Could you check a few things on this model? Use its own coordinates, in mm. Face numbers are marked on the shaded views. Round coordinates to 2 decimals unless told otherwise and drop trailing zeros. Answer in a Markdown table with one row per item.
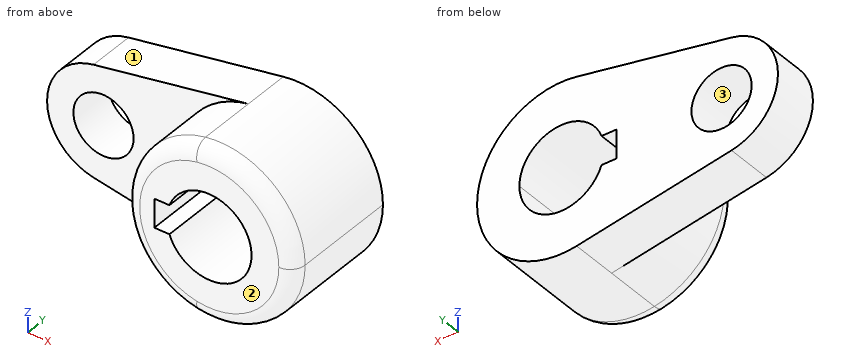
from build123d import *

# Parameters (mm, degrees)
F1_DEPTH = 40.1828
F2_DEPTH = 15.7734
F0_R     = 10.16
F3_DEPTH = 15.7734
F4_R     = 5.08


with BuildPart() as f1:
    # F0 (on Front) → F1 (new body)
    with BuildSketch(Plane.XZ):
        with BuildLine():
            ThreePointArc((-5.042647, -28.126541), (18.336262, -21.916025), (28.575, 0))
            ThreePointArc((28.575, 0), (18.336262, 21.916025), (-5.042647, 28.126541))
            ThreePointArc((-5.042647, 28.126541), (-28.575, 0), (-5.042647, -28.126541))
        make_face()
        with BuildLine():
            ThreePointArc((-13.447765, 4.826), (2.449257, 14.076001), (14.2875, 0))
            ThreePointArc((14.2875, 0), (2.449257, -14.076001), (-13.447765, -4.826))
            Line((-13.447765, -4.826), (-18.5293, -4.826))
            Line((-18.5293, -4.826), (-18.5293, 4.826))
            Line((-18.5293, 4.826), (-13.447765, 4.826))
        make_face(mode=Mode.SUBTRACT)
    extrude(amount=F1_DEPTH)

    # F0 (on Front) → F2 (join)
    with BuildSketch(Plane.XZ):
        with BuildLine():
            ThreePointArc((-5.042647, -28.126541), (-28.575, 0), (-5.042647, 28.126541))
            Line((-5.042647, 28.126541), (-57.336765, 18.751028))
            ThreePointArc((-57.336765, 18.751028), (-41.750826, 14.610683), (-34.925, 0))
            ThreePointArc((-34.925, 0), (-41.750826, -14.610683), (-57.336765, -18.751028))
            Line((-57.336765, -18.751028), (-5.042647, -28.126541))
        make_face()
    extrude(amount=F2_DEPTH)

    # F0 (on Front) → F3 (join)
    with BuildSketch(Plane.XZ):
        with BuildLine():
            ThreePointArc((-34.925, 0), (-41.750826, 14.610683), (-57.336765, 18.751028))
            ThreePointArc((-57.336765, 18.751028), (-73.025, 0), (-57.336765, -18.751028))
            ThreePointArc((-57.336765, -18.751028), (-41.750826, -14.610683), (-34.925, 0))
        make_face()
        with Locations((-53.975, 0)):
            Circle(F0_R, mode=Mode.SUBTRACT)
    extrude(amount=F3_DEPTH)

    # F4
    f4_edges = [f1.edges().sort_by_distance(p)[0] for p in [
        (-28.575, -40.1828, 0),
    ]]
    fillet(f4_edges, radius=F4_R)


solid = f1.part
1) Please list where these lines run through material, in increasing order: line 1 (Y direction, x = -33, z = -8); line 2 (X direction, y = -20, z = 3.5); line 3 (Z direction, x = -47, y = -6.5).
Findings:
| item | result |
|---|---|
| line 1 | y = -15.77 to 0 |
| line 2 | x = -28.36 to -18.53, 13.85 to 28.36 |
| line 3 | z = -20.6 to -7.39, 7.39 to 20.6 |
2) For pin 1 (8 mm diameter, centred on y = -25, z = -14.5, fed in from -X); pin 2 (2 mm diameter, centred on y = -16.5, z = 13, fed in from +X); pin 3 (5.5 mm diameter, centred on x = -16.5, y = -19, fed in from -Z), each with a flat end and sliding along its axis, tell me the tip position at first contact or that it passes through.
Findings:
| item | result |
|---|---|
| pin 1 | stops at x = -26.58 |
| pin 2 | stops at x = 25.93 |
| pin 3 | stops at z = -25.05 |
3) Thinking about a two-plate mould opening in X: for the marked faces 1, 2 and 3, which applies, +X half, -X half, draft (parallel to the pull), parting line (faces both ways), or undercut?
Findings:
| item | result |
|---|---|
| face 1 | -X half |
| face 2 | draft |
| face 3 | undercut |
4) Imagine slicing it at B-B, the plane y = -8.5. Count the separate pieces of the cut face and the enclosed holes in it, plus the area to 3 significant figures.
Findings:
| item | result |
|---|---|
| separate pieces | 1 |
| enclosed holes | 2 |
| area | 3,450 mm^2 |
